from build123d import *

# Parameters (mm, degrees)
ESQUISSE1_R             = 2
ESQUISSE1_R_2           = 1.5
BOSS_EXTRU_1_DEPTH      = 3
BOSS_EXTRU_2_START      = -3
ESQUISSE3_R             = 7.5
BOSS_EXTRU_2_DEPTH      = 6
ESQUISSE4_R             = 3.875
ENL_V_MAT_EXTRU_1_DEPTH = 1
ESQUISSE5_R             = 2.375
ENL_V_MAT_EXTRU_2_DEPTH = 4


with BuildPart() as part:
    # Esquisse1 → Boss.-Extru.1 (new body)
    with BuildSketch(Plane.XY):
        Polygon((-61.381557247, 0), (61.381557247, 0), (61.381557247, -45.5212086), (25, -45.5212086), (25, -80), (-25, -80), (-25, -45.5212086), (-61.381557247, -45.5212086), align=None)
        with Locations((0, -20)):
            Circle(ESQUISSE1_R, mode=Mode.SUBTRACT)
        with Locations((-20, -55)):
            Circle(ESQUISSE1_R_2, mode=Mode.SUBTRACT)
        with Locations((20, -55)):
            Circle(ESQUISSE1_R_2, mode=Mode.SUBTRACT)
        with Locations((20, -75)):
            Circle(ESQUISSE1_R_2, mode=Mode.SUBTRACT)
        with Locations((-20, -75)):
            Circle(ESQUISSE1_R_2, mode=Mode.SUBTRACT)
        with Locations((56.381557247, -40.5212086)):
            Circle(ESQUISSE1_R, mode=Mode.SUBTRACT)
        with Locations((-56.381557247, -40.5212086)):
            Circle(ESQUISSE1_R, mode=Mode.SUBTRACT)
    extrude(amount=BOSS_EXTRU_1_DEPTH)

    # Esquisse3 → Boss.-Extru.2 (add)
    with BuildSketch(Plane(origin=(0, 0, 0), x_dir=(-1, 0, 0), z_dir=(0, 0, -1)).offset(BOSS_EXTRU_2_START)):
        with Locations((56.381557247, -40.5212086)):
            Circle(ESQUISSE3_R)
        with Locations((0, -20)):
            Circle(ESQUISSE3_R)
    extrude(amount=BOSS_EXTRU_2_DEPTH)

    # Esquisse4 → Enlèv. mat.-Extru.1 (cut)
    with BuildSketch(Plane(origin=(0, 0, -3), x_dir=(-1, 0, 0), z_dir=(0, 0, -1))):
        with Locations((56.381557247, -40.5212086)):
            Circle(ESQUISSE4_R)
        with Locations((0, -20)):
            Circle(ESQUISSE4_R)
    extrude(amount=-ENL_V_MAT_EXTRU_1_DEPTH, mode=Mode.SUBTRACT)

    # Esquisse5 → Enlèv. mat.-Extru.2 (cut)
    with BuildSketch(Plane(origin=(0, 0, -2), x_dir=(-1, 0, 0), z_dir=(0, 0, -1))):
        with Locations((56.381557247, -40.5212086)):
            Circle(ESQUISSE5_R)
        with Locations((0, -20)):
            Circle(ESQUISSE5_R)
    extrude(amount=-ENL_V_MAT_EXTRU_2_DEPTH, mode=Mode.SUBTRACT)


solid = part.part
Input: part model. Units: mm. Frame: model coordinates. A direction names the side the tool comes from. Coordinates: 2 decimals unless noted, no trailing zeros. Write each loop counter-clockwise with the first axis right and the second up, starting at its lowest first coordinate (ties: lowest second). Pieces come first, ordered by that corner, then holes. Notation, with made-up numbers: M -2,-13.5 L 51,-13.5 A24 ccw 51,12.5 Z; hole C -29.5,-2 d11. An arc over 180 degrees is marked long. Answer as a JSON object with one key per item and string values. Group by question number.
(1) Contact query for flat-ended pins moving along their axis: P1, Ø4.5, axis at x = 0, y = -20, coming from the -Z side; P2, Ø2, axis at y = -26, z = -0.5, coming from the -X side; P3, Ø24, axis at x = -11, y = -52, coming from the -Z side; P4, Ø1.5, axis at y = -59.5, z = -1, coming from the +X side. Output: stop coordinate, or through.
(2) Ray query, line 1 along Y through (x, z) = (20, 1.4); line 2 along X through (y, z) = (-75, 1.05); line 3 along Y through (x, z) = (21, 2.05). Return the intervals inside material, ascending. Write a range as [from, to].
(3) Section B-B on x = 20. Output: boundary loops of the cut face in (y, z), plus the area to 3 significant figures.
(4) Section A-A on y = -55. Output: boundary loops of the cut face in (x, z).
(5) Mould query, pull axis X, two halves, no side actions, for faces 5 (the face through (61.382, -22, 1)), 6 (the face through (-20.195, -73.513, 1.479)), 7 (the face through (1, -31, 0)). Classes: pulls with the +X half, pulls with the -X half, needs draft (parallel to the pull), parting line crosses it, or undercut.
(6) Section D-D on x = -36.5. Output: boundary loops of the cut face in (y, z), plus the area to 3 significant figures.
(7) Set-up query: faces 1 (the face through (43, -45.521, 1)), 2 (the face through (0.504, -16.158, -2.507)), 3 (the face through (-38, -45.521, 1)), 4 (the face through (-61.382, -18, 1)). Return all of +Z, -Z, +X, -X, +Y, -Y with unobstructed straight access to the full face (end or side cutting, diameter ignored); none if empty.
(8) Section C-C on y = -20. Output: boundary loops of the cut face in (x, z) (3 decimals), plus the area to 3 significant figures.
Result set:
{
 "1": {"P1": "stops at z = 2", "P2": "stops at x = -61.38", "P3": "stops at z = 0", "P4": "passes through"},
 "2": {"line 1": "y = [-80, -76.5], [-73.5, -56.5], [-53.5, 0]", "line 2": "x = [-25, -21.5], [-18.5, 18.5], [21.5, 25]", "line 3": "y = [-80, -76.12], [-73.88, -56.12], [-53.88, 0]"},
 "3": {"outline": "M -80,0 L -76.5,0 L -76.5,3 L -80,3 Z; M -73.5,0 L -56.5,0 L -56.5,3 L -73.5,3 Z; M -53.5,0 L 0,0 L 0,3 L -53.5,3 Z", "area": "222 mm2"},
 "4": {"outline": "M -25,0 L -21.5,0 L -21.5,3 L -25,3 Z; M -18.5,0 L 18.5,0 L 18.5,3 L -18.5,3 Z; M 21.5,0 L 25,0 L 25,3 L 21.5,3 Z"},
 "5": {"face 5": "pulls with the +X half", "face 6": "undercut", "face 7": "needs draft"},
 "6": {"outline": "M -45.52,0 L 0,0 L 0,3 L -45.52,3 Z", "area": "137 mm2"},
 "7": {"face 1": "+Z, -Z, +X, -Y", "face 2": "-Z", "face 3": "+Z, -Z, -Y", "face 4": "+Z, -Z, -X, +Y"},
 "8": {"outline": "M -61.382,0 L -7.5,0 L -7.5,-3 L -3.875,-3 L -3.875,-2 L -2.375,-2 L -2.375,2 L 2.375,2 L 2.375,-2 L 3.875,-2 L 3.875,-3 L 7.5,-3 L 7.5,0 L 61.382,0 L 61.382,3 L -61.382,3 Z", "area": "387 mm2"}
}
